The listing builds one solid part. Answer for the finished solid, in the listing's coordinates (mm). A direction names the side the tool comes from. Round coordinates to 2 decimals unless told otherwise and drop trailing zeros. Loops run counter-clockwise (first coordinate to the right, second up) from the corner with the lowest first, then second, coordinate; pieces in that order, holes last. Notation, with made-up numbers: M 5.25,-40 L 50.25,-40 A13 ccw 50.25,-25 Z; hole C 82,84 d2. An arc over 180 degrees is marked long. Answer as a JSON object with one key per item and string values.
```python
from build123d import *

# Parameters (mm, degrees)
CROQUIS1_W              = 80
CROQUIS1_H              = 36
CROQUIS1_R              = 1.25
SALIENTE_EXTRUIR2_DEPTH = 1.6
CROQUIS2_W              = 71.3
CROQUIS2_H              = 26.3
SALIENTE_EXTRUIR3_DEPTH = 4.6
CROQUIS3_W              = 64.5
CROQUIS3_H              = 16.4
CORTAR_EXTRUIR1_DEPTH   = 1
CROQUIS5_R              = 1
SALIENTE_EXTRUIR4_DEPTH = 32
REVOLUCI_N3_ANGLE       = 90


with BuildPart() as part:
    # Croquis1 → Saliente-Extruir2 (new body)
    with BuildSketch(Plane.XY):
        with Locations((40, 18)):
            Rectangle(CROQUIS1_W, CROQUIS1_H)
        with Locations((77.5, 33.5)):
            Circle(CROQUIS1_R, mode=Mode.SUBTRACT)
        with Locations((77.5, 2.5)):
            Circle(CROQUIS1_R, mode=Mode.SUBTRACT)
        with Locations((2.5, 2.5)):
            Circle(CROQUIS1_R, mode=Mode.SUBTRACT)
        with Locations((2.5, 33.5)):
            Circle(CROQUIS1_R, mode=Mode.SUBTRACT)
    extrude(amount=SALIENTE_EXTRUIR2_DEPTH)

    # Croquis2 → Saliente-Extruir3 (add)
    with BuildSketch(Plane.XY.offset(1.6)):
        with Locations((40, 18)):
            Rectangle(CROQUIS2_W, CROQUIS2_H)
    extrude(amount=SALIENTE_EXTRUIR3_DEPTH)

    # Croquis3 → Cortar-Extruir1 (cut)
    with BuildSketch(Plane.XY.offset(6.2)):
        with Locations((40, 18)):
            Rectangle(CROQUIS3_W, CROQUIS3_H)
    extrude(amount=-CORTAR_EXTRUIR1_DEPTH, mode=Mode.SUBTRACT)

    # Croquis5 → Saliente-Extruir4 (add, symmetric)
    with BuildSketch(Plane(origin=(40, 0, 0), x_dir=(0, 0, -1), z_dir=(1, 0, 0))):
        with Locations((-6.2, 28.675)):
            Circle(CROQUIS5_R)
        with Locations((-6.2, 7.325)):
            Circle(CROQUIS5_R)
    extrude(amount=SALIENTE_EXTRUIR4_DEPTH, both=True)

    # Croquis4 → Revolución3 (revolve)
    with BuildSketch(Plane.XY.offset(6.2)):
        with BuildLine():
            Line((72, 29.675), (72, 27.675))
            ThreePointArc((72, 27.675), (73, 28.675), (72, 29.675))
        make_face()
    revolve(axis=Axis((72, 29.675, 6.2), (0, -1, 0)), revolution_arc=REVOLUCI_N3_ANGLE)

    # Croquis6 → Revolución4 (revolve)
    with BuildSketch(Plane.XY.offset(6.2)):
        with BuildLine():
            Line((8, 29.675), (8, 27.675))
            ThreePointArc((8, 27.675), (7, 28.675), (8, 29.675))
        make_face()
    revolve(axis=Axis((8, 29.675, 6.2), (0, -1, 0)))

    # Croquis7 → Revolución5 (revolve)
    with BuildSketch(Plane.XY.offset(6.2)):
        with BuildLine():
            Line((8, 8.325), (8, 6.325))
            ThreePointArc((8, 6.325), (7, 7.325), (8, 8.325))
        make_face()
    revolve(axis=Axis((8, 8.325, 6.2), (0, -1, 0)))

    # Croquis8 → Revolución6 (revolve)
    with BuildSketch(Plane.XY.offset(6.2)):
        with BuildLine():
            Line((72, 8.325), (72, 6.325))
            ThreePointArc((72, 6.325), (73, 7.325), (72, 8.325))
        make_face()
    revolve(axis=Axis((72, 8.325, 6.2), (0, -1, 0)))


solid = part.part
```
Item 1: Which of the six approach directions +Z, -Z, +X, -X, +Y, -Y give full straight-line access (tool end or side, diameter ignored) to faces 4 (the face through (40, 18, 5.2)), 5 (the face through (40, 31.15, 4)), 6 (the face through (40, 4.85, 4)), 7 (the face through (75.65, 18, 4))?
Values follow:
{"face 4": "+Z", "face 5": "+Z, +X, -X, +Y", "face 6": "+Z, +X, -X, -Y", "face 7": "+Z, +X, +Y, -Y"}
Item 2: The part is cut by section D-D (y = 24.5). Give the vertices of the cut face in (x, z), then the cut area to 3 significant figures.
Values follow:
{"outline": "M 0,0 L 80,0 L 80,1.6 L 75.65,1.6 L 75.65,6.2 L 72.25,6.2 L 72.25,5.2 L 7.75,5.2 L 7.75,6.2 L 4.35,6.2 L 4.35,1.6 L 0,1.6 Z", "area": "391 mm^2"}
Item 3: The part is cut by section B-B (x = 77.5). Give the vertices of the cut face in (y, z), then the cut area to 3 significant figures.
Values follow:
{"outline": "M 0,0 L 1.25,0 L 1.25,1.6 L 0,1.6 Z; M 3.75,0 L 32.25,0 L 32.25,1.6 L 3.75,1.6 Z; M 34.75,0 L 36,0 L 36,1.6 L 34.75,1.6 Z", "area": "49.6 mm^2"}
Item 4: Determine the mould class of faces 1 (the face through (78.655, 33.021, 0.789)), 2 (the face through (42, 27, 6.2)), 3 (the face through (4.35, 18, 4)) for opening direction X: released by +X, released by -X, zero draft, split by the parting line, or undercut.
Values follow:
{"face 1": "undercut", "face 2": "zero draft", "face 3": "released by -X"}
Item 5: Straight lines are drawn through the part: line 1 (Y direction, x = 77.5, z = 1.35); line 2 (Y direction, x = 4.5, z = 3.5); line 3 (Z direction, x = 54, y = 25). For each, find the intervals that lie inside material, in ascending order.
Values follow:
{"line 1": "0 to 1.25, 3.75 to 32.25, 34.75 to 36", "line 2": "4.85 to 31.15", "line 3": "0 to 5.2"}
Item 6: Flat-ended cylindrical pins translate along their axes: P1, Ø5, axis at x = 39.5, y = 13.5, coming from the +Z side; P2, Ø3.5, axis at x = 55, z = 5, coming from the +Y side; P3, Ø2, axis at x = 2.5, y = 2.5, coming from the -Z side; P4, Ø3.5, axis at y = 21.5, z = 4, coming from the +X side. Find the tip coordinate at first contact, or state that the pin passes through.
Values follow:
{"P1": "z = 5.2", "P2": "y = 31.15", "P3": "through", "P4": "x = 75.65"}
Item 7: The part is cut by section C-C (x = 63). Give the vertices of the cut face in (y, z) (3 decimals), then the cut area to 3 significant figures.
Values follow:
{"outline": "M 0,0 L 36,0 L 36,1.6 L 31.15,1.6 L 31.15,6.2 L 29.675,6.2 A1 ccw 27.675,6.2 L 26.2,6.2 L 26.2,5.2 L 9.8,5.2 L 9.8,6.2 L 8.325,6.2 A1 ccw 6.325,6.2 L 4.85,6.2 L 4.85,1.6 L 0,1.6 Z", "area": "165 mm^2"}
Item 8: The part is cut by section A-A (y = 33.5). Give the vertices of the cut face in (x, z), then the cut area to 3 significant figures.
Values follow:
{"outline": "M 0,0 L 1.25,0 L 1.25,1.6 L 0,1.6 Z; M 3.75,0 L 76.25,0 L 76.25,1.6 L 3.75,1.6 Z; M 78.75,0 L 80,0 L 80,1.6 L 78.75,1.6 Z", "area": "120 mm^2"}
